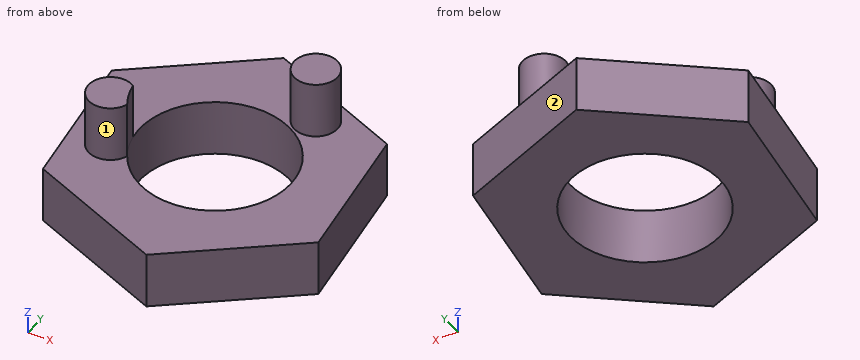
```python
from build123d import *

# Parameters (mm, degrees)
F0_R     = 33.4292406747
F1_DEPTH = 25
F2_R     = 9.6236756303
F3_DEPTH = 25


# Not quite as in the source:
# - after a boolean that leaves OpenCascade's solid faulty, fix() repairs it


with BuildPart() as f1:
    # F0 (on Top) → F1 (new body)
    with BuildSketch(Plane.XY):
        Polygon((-8.0187594833, 61.3087737227), (-60.6567287502, 21.6589621043), (-52.6379692669, -43.7517622936), (8.0187594833, -69.5126750732), (60.6567287502, -29.8628634548), (52.6379692669, 35.5478609431), align=None)
        with Locations((0, -4.1019506752)):
            Circle(F0_R, mode=Mode.SUBTRACT)
    extrude(amount=F1_DEPTH)

    # F2 (on face) → F3 (join)
    with BuildSketch(Plane.XY.offset(25)):
        with BuildLine():
            ThreePointArc((-28.942967923, -20.8297341476), (-31.4616986723, -15.4013156461), (-32.9722113693, -9.6107989674))
            ThreePointArc((-32.9722113693, -9.6107989674), (-47.2113068424, -21.0577353047), (-28.942967923, -20.8297341476))
        make_face()
        with Locations((22.0662225038, 34.1823846102)):
            Circle(F2_R)
    extrude(amount=F3_DEPTH)

    add(f1.part.fix(), mode=Mode.REPLACE)


solid = f1.part
```
Could you check a few things on this model? Use its own coordinates, in mm. Face numbers are marked on the shaded views. A direction names the side the tool comes from. Round coordinates to 2 decimals unless told otherwise and drop trailing zeros. Loops run counter-clockwise (first coordinate to the right, second up) from the corner with the lowest first, then second, coordinate; pieces in that order, holes last. Notation, with made-up numbers: (-7.5, 19) -> (16.5, 19) arc R9 cw to (16.5, 36) -> close; hole circle Ø1 at (0, -34.5). An arc over 180 degrees is marked (long way). Put each result on its own line as item: value.
Q1. I want a section at A-A on y = -6.5. Write out the boundary of the cut face in (x, z), and give its area (3 significant figures).
Checks:
outline: (-57.2, 0) -> (-33.34, 0) -> (-33.34, 25) -> (-57.2, 25) -> close; (33.34, 0) -> (57.79, 0) -> (57.79, 25) -> (33.34, 25) -> close
area: 1,210 mm2
Q2. For pin 1 Ø1.5 at (x, y) = (-30.5, 2) entering from +Z; pin 2 Ø4 at (x, z) = (48, 24.5) entering from -Y; pin 3 Ø5 at (x, z) = (-43, 22.5) entering from -Y; pin 4 Ø2 at (y, z) = (15.5, 16.5) entering from +X, each with a flat end and sliding along its axis, tell me the tip position at first contact or that it passes through.
Checks:
pin 1: through
pin 2: y = -40.9
pin 3: y = -48.91
pin 4: x = 55.22
Q3. I want a section at D-D on x = 26. Write out the boundary of the cut face in (y, z), and give its area (3 significant figures).
Checks:
outline: (-55.97, 0) -> (-25.11, 0) -> (-25.11, 25) -> (-55.97, 25) -> close; (16.91, 0) -> (46.86, 0) -> (46.86, 25) -> (42.97, 25) -> (42.97, 50) -> (25.4, 50) -> (25.4, 25) -> (16.91, 25) -> close
area: 1,960 mm2
Q4. I want a section at B-B on x = 0. Write out the boundary of the cut face in (y, z).
Checks:
outline: (-66.11, 0) -> (-37.53, 0) -> (-37.53, 25) -> (-66.11, 25) -> close; (29.33, 0) -> (57.9, 0) -> (57.9, 25) -> (29.33, 25) -> close
Q5. Which directions (+Z, -Z, +X, -X, +Y, -Y) give clear straight access to the entire face, cutting with the end or side of a thin tool? Please do the marked faces 1 and 2.
Checks:
face 1: +Z
face 2: +Z, -Z, +X, +Y
Q6. Please list where these lines run through material, in increasing order: line 1 (Z direction, x = -11, y = 50); line 2 (Y direction, x = 0, z = 7.5); line 3 (Y direction, x = -30, z = 10). Write a range as from..to.
Checks:
line 1: 0..25
line 2: -66.11..-37.53, 29.33..57.9
line 3: -53.37..-18.85, 10.65..44.75
Q7. I want a section at C-C on z = 21. Write out the boundary of the cut face in (x, y), and give its area (3 significant figures).
Checks:
outline: (-60.66, 21.66) -> (-52.64, -43.75) -> (8.02, -69.51) -> (60.66, -29.86) -> (52.64, 35.55) -> (-8.02, 61.31) -> close; hole circle Ø66.86 at (0, -4.1)
area: 7,770 mm2
